Source: CAD feature listing. Evaluate the final solid. Frame: model axes, mm. Round coordinates to 2 decimals unless told otherwise and drop trailing zeros. Order: outer loops, then holes, each group sorted by start corner. A loop starts at its lowest first (then second) coordinate and runs counter-clockwise, first axis right, second up. Notation, with made-up numbers: (37, -11.75) -> (74, -11.75) arc R19 cw to (74, 20.25) -> close; hole circle Ø5 at (28, -30). An arc over 180 degrees is marked (long way). Use a Markdown table: item, result. Add a question column.
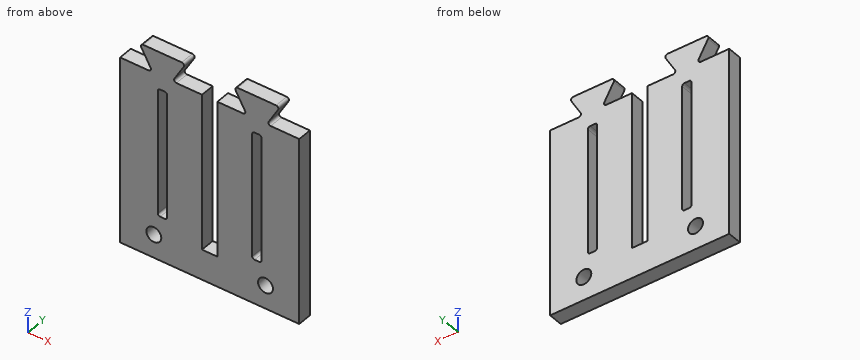
```python
from build123d import *

# Parameters (mm, degrees)
BOSS_EXTRUDE1_DEPTH         = 3.05
FILLET1_R                   = 0.5
SKETCH3_W                   = 3.3
SKETCH3_H                   = 61.8
SKETCH3_H_2                 = 1
CUT_EXTRUDE2_DEPTH          = 45.495673947
SKETCH8_W                   = 2
SKETCH8_H                   = 27.5
CUT_EXTRUDE3_DEPTH          = 45.495673947
FILLET2_R                   = 0.5
M3_CLEARANCE_DAMPER_HOLES_D = 3.2


with BuildPart() as part:
    # Sketch1 → Boss-Extrude1 (new body)
    with BuildSketch(Plane(origin=(0, 0, 0), x_dir=(1, 0, 0), z_dir=(0, 1, 0))):
        Polygon((-19.25, 0), (-19.25, 40), (19.25, 40), (19.25, 0), (12.25, 0), (15.136751346, -5), (5.136751346, -5), (8.023502692, 0), (-8.023502692, 0), (-5.136751346, -5), (-15.136751346, -5), (-12.25, 0), align=None)
    extrude(amount=BOSS_EXTRUDE1_DEPTH)

    # Fillet1
    fillet1_edges = [part.edges().sort_by_distance(p)[0] for p in [
        (12.25, 1.525, 0),
        (15.136751346, 1.525, 5),
        (5.136751346, 1.525, 5),
        (8.023502692, 1.525, 0),
        (-8.023502692, 1.525, 0),
        (-5.136751346, 1.525, 5),
        (-15.136751346, 1.525, 5),
        (-12.25, 1.525, 0),
    ]]
    fillet(fillet1_edges, radius=FILLET1_R)

    # Sketch3 → Cut-Extrude2 (cut, through all)
    with BuildSketch(Plane(origin=(0, 3.05, 0), x_dir=(1, 0, 0), z_dir=(0, 1, 0))):
        with Locations((0, 2.6)):
            Rectangle(SKETCH3_W, SKETCH3_H)
        with Locations((0, -30)):
            Rectangle(SKETCH3_W, SKETCH3_H_2)
    extrude(amount=-CUT_EXTRUDE2_DEPTH, mode=Mode.SUBTRACT)

    # Sketch8 → Cut-Extrude3 (cut, through all)
    with BuildSketch(Plane(origin=(0, 3.05, 0), x_dir=(1, 0, 0), z_dir=(0, 1, 0))):
        with Locations((-10.136751346, 16.75)):
            Rectangle(SKETCH8_W, SKETCH8_H)
        with Locations((10.136751346, 16.75)):
            Rectangle(SKETCH8_W, SKETCH8_H)
    extrude(amount=-CUT_EXTRUDE3_DEPTH, mode=Mode.SUBTRACT)

    # Fillet2
    fillet2_edges = [part.edges().sort_by_distance(p)[0] for p in [
        (-11.136751346, 1.525, -3),
        (-11.136751346, 1.525, -30.5),
        (-9.136751346, 1.525, -30.5),
        (-9.136751346, 1.525, -3),
        (11.136751346, 1.525, -30.5),
        (11.136751346, 1.525, -3),
        (9.136751346, 1.525, -3),
        (9.136751346, 1.525, -30.5),
    ]]
    fillet(fillet2_edges, radius=FILLET2_R)

    # M3 Clearance Damper Holes (through all)
    with Locations(Plane(origin=(0, 3.05, 0), x_dir=(1, 0, 0), z_dir=(0, 1, 0))):
        with Locations((-12, 35), (12, 35)):
            Hole(M3_CLEARANCE_DAMPER_HOLES_D / 2)


solid = part.part
```
1) First-contact query: pin 1 Ø12 at (x, z) = (-2, -25.5) entering from -Y. Flat tip, straight axial feed; report the tip coordinate or a pass-through.
2) Section C-C on z = -32. Output: boundary loops of the cut face in (x, y), then the cut area to 3 significant figures.
3) Section B-B on x = 12. Output: boundary loops of the cut face in (y, z).
4) Line query: probe 1 along X at (y, z) = (1.25, -35); probe 2 along X at (y, z) = (2.75, -19). Output: solid intervals per line, ascending. Write a range as from..to.
5) Section D-D on y = 0.95. Count the separate pieces of the cut face and the enclosed holes in it, then the cut area to 3 significant figures.
6) Section A-A on z = -18.5. Output: boundary loops of the cut face in (x, y), then the cut area to 3 significant figures.
Conclusion:
| question | item | result |
|---|---|---|
| 1 | pin 1 | stops at y = 0 |
| 2 | outline | (-19.25, 0) -> (-1.65, 0) -> (-1.65, 3.05) -> (-19.25, 3.05) -> close; (1.65, 0) -> (19.25, 0) -> (19.25, 3.05) -> (1.65, 3.05) -> close |
| 2 | area | 107 mm^2 |
| 3 | outline | (0, -40) -> (3.05, -40) -> (3.05, -36.6) -> (0, -36.6) -> close; (0, -33.4) -> (3.05, -33.4) -> (3.05, 5) -> (0, 5) -> close |
| 4 | probe 1 | x = -19.25..-13.6, -10.4..10.4, 13.6..19.25 |
| 4 | probe 2 | x = -19.25..-11.14, -9.14..-1.65, 1.65..9.14, 11.14..19.25 |
| 5 | separate pieces | 1 |
| 5 | enclosed holes | 4 |
| 5 | area | 1,370 mm^2 |
| 6 | outline | (-19.25, 0) -> (-11.14, 0) -> (-11.14, 3.05) -> (-19.25, 3.05) -> close; (-9.14, 0) -> (-1.65, 0) -> (-1.65, 3.05) -> (-9.14, 3.05) -> close; (1.65, 0) -> (9.14, 0) -> (9.14, 3.05) -> (1.65, 3.05) -> close; (11.14, 0) -> (19.25, 0) -> (19.25, 3.05) -> (11.14, 3.05) -> close |
| 6 | area | 95.2 mm^2 |
